Source: CAD feature listing. Evaluate the final solid. Frame: model axes, mm. Face numbers are marked on the shaded views. A direction names the side the tool comes from. Round coordinates to 2 decimals unless told otherwise and drop trailing zeros. Write each loop counter-clockwise with the first axis right and the second up, starting at its lowest first coordinate (ties: lowest second). Pieces come first, ordered by that corner, then holes.
from build123d import *

# Parameters (mm, degrees)
F0_R     = 15
F0_R_2   = 6
F0_R_3   = 4
F1_DEPTH = 60
F2_DEPTH = 180
F3_DEPTH = 160


with BuildPart() as f1:
    # F0 (on Right) → F1 (new body)
    with BuildSketch(Plane.YZ):
        Circle(F0_R)
        Circle(F0_R_2, mode=Mode.SUBTRACT)
        Circle(F0_R_2)
        Circle(F0_R_3, mode=Mode.SUBTRACT)
        Circle(F0_R_3)
    extrude(amount=F1_DEPTH)

    # F0 (on Right) → F2 (join)
    with BuildSketch(Plane.YZ):
        Circle(F0_R_2)
        Circle(F0_R_3, mode=Mode.SUBTRACT)
    extrude(amount=F2_DEPTH)

    # F0 (on Right) → F3 (join)
    with BuildSketch(Plane.YZ):
        Circle(F0_R_3)
    extrude(amount=F3_DEPTH)


solid = f1.part
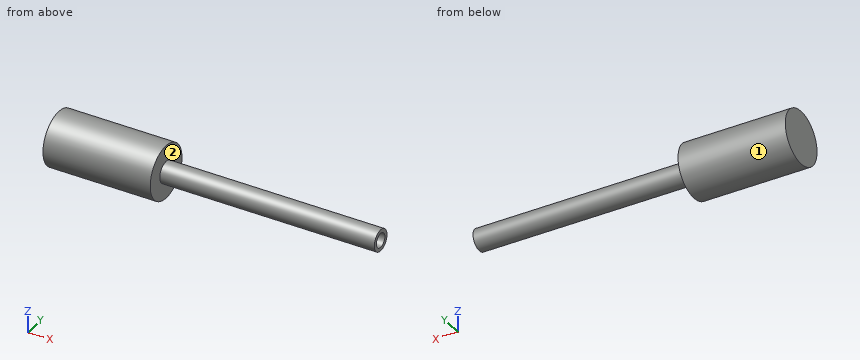
1) Reachability of the marked faces 1 and 2 from +Z, -Z, +X, -X, +Y, -Y: full face, straight path, thin tool, end or side. Return the list, or none.
Taken from the geometry:
face 1: +X, -X
face 2: +X
2) Section query C-C on x = 169.5. Return the cut outline in (y, z), then the cut area to 3 significant figures.
Taken from the geometry:
outline: circle Ø12 at (0, 0); hole circle Ø8 at (0, 0)
area: 62.8 mm2
3) Material intervals for line 1 (Z direction, x = 172.5, y = 0); line 2 (X direction, y = -2.5, z = -9.75); line 3 (X direction, y = 1.75, z = -0.25), sorted ascending.
Taken from the geometry:
line 1: z = -6 to -4, 4 to 6
line 2: x = 0 to 60
line 3: x = 0 to 160
4) Section query A-A on z = 0. Return the cut outline in (x, y), then the cut area to 3 significant figures.
Taken from the geometry:
outline: (0, -15) - (60, -15) - (60, -6) - (180, -6) - (180, -4) - (160, -4) - (160, 4) - (180, 4) - (180, 6) - (60, 6) - (60, 15) - (0, 15) - close
area: 3,080 mm2
5) Section query D-D on x = 68. Return the cut outline in (y, z).
Taken from the geometry:
outline: circle Ø12 at (0, 0)
6) Contact query for flat-ended pins moving along their axis: P1, Ø8, axis at x = 37.5, z = -11.5, coming from the +Y side; P2, Ø7, axis at y = 0, z = 0, coming from the +X side; P3, Ø2, axis at y = 1, z = -11, coming from the +X side. Output: stop coordinate, or through.
Taken from the geometry:
P1: stops at y = 12.99
P2: stops at x = 160
P3: stops at x = 60
